Could you check a few things on this model? Use its own coordinates, in mm. Face numbers are marked on the shaded views. A direction names the side the tool comes from. Give positions to 0.01 mm unless a question says otherwise; leave off trailing zeros. Loops run counter-clockwise (first coordinate to the right, second up) from the corner with the lowest first, then second, coordinate; pieces in that order, holes last. Notation, with made-up numbers: (21, -8) -> (63, -8) arc R19 cw to (63, 24) -> close; hole circle Ø2 at (24, 27.25). An arc over 180 degrees is marked (long way). Put each result on its own line as item: value.
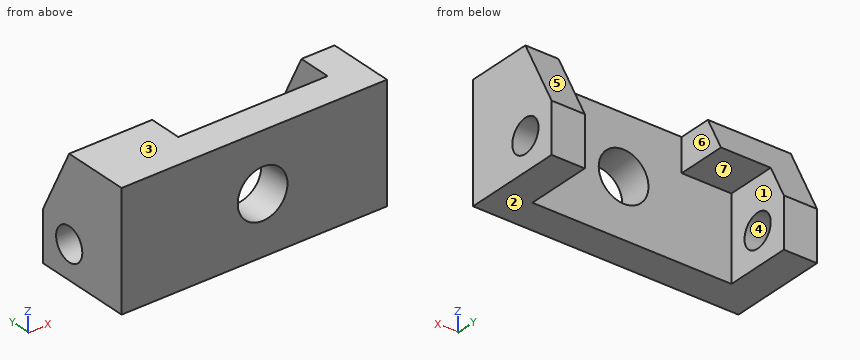
```python
from build123d import *

# Parameters (mm, degrees)
SKETCH1_W           = 80
SKETCH1_H           = 35
BOSS_EXTRUDE1_DEPTH = 30
CUT_EXTRUDE1_DEPTH  = 20
CUT_EXTRUDE2_DEPTH  = 81
SKETCH4_R           = 5
CUT_EXTRUDE4_DEPTH  = 81
SKETCH5_R           = 7.5
CUT_EXTRUDE5_DEPTH  = 11


with BuildPart() as part:
    # Sketch1 → Boss-Extrude1 (new body)
    with BuildSketch(Plane(origin=(0, 0, 0), x_dir=(1, 0, 0), z_dir=(0, 1, 0))):
        with Locations((40, 17.5)):
            Rectangle(SKETCH1_W, SKETCH1_H)
    extrude(amount=BOSS_EXTRUDE1_DEPTH)

    # Sketch2 → Cut-Extrude1 (cut)
    with BuildSketch(Plane(origin=(0, 30, 0), x_dir=(1, 0, 0), z_dir=(0, 1, 0))):
        Polygon((10, 35), (10, 10.002355001), (25, 10.002355001), (25, 0), (70, 0), (70, 35), align=None)
    extrude(amount=-CUT_EXTRUDE1_DEPTH, mode=Mode.SUBTRACT)

    # Sketch3 → Cut-Extrude2 (cut, through all)
    with BuildSketch(Plane.ZY):
        Polygon((0, 30), (0, 20), (-20, 30), align=None)
    extrude(amount=-CUT_EXTRUDE2_DEPTH, mode=Mode.SUBTRACT)

    # Sketch4 → Cut-Extrude4 (cut, through all)
    with BuildSketch(Plane(origin=(80, 0, 0), x_dir=(0, 0, -1), z_dir=(1, 0, 0))):
        with Locations((25, 20)):
            Circle(SKETCH4_R)
    extrude(amount=-CUT_EXTRUDE4_DEPTH, mode=Mode.SUBTRACT)

    # Sketch5 → Cut-Extrude5 (cut, through all)
    with BuildSketch(Plane(origin=(0, 10, 0), x_dir=(1, 0, 0), z_dir=(0, 1, 0))):
        with Locations((42.5, 17.5)):
            Circle(SKETCH5_R)
    extrude(amount=-CUT_EXTRUDE5_DEPTH, mode=Mode.SUBTRACT)


solid = part.part
```
1. If we section it at A-A (x = 48.5): List the corners of the cut face in (y, z) for me, then the cut area to 3 significant figures.
Recorded:
outline: (0, -35) -> (10, -35) -> (10, -22) -> (0, -22) -> close; (0, -13) -> (10, -13) -> (10, 0) -> (0, 0) -> close
area: 260 mm^2
2. I'm going to push flat-ended pins straight in: pin 1 (6 mm diameter, centred on x = 70.5, z = -30.5, fed in from -Y); pin 2 (5 mm diameter, centred on x = 48, z = -8, fed in from +Y); pin 3 (10 mm diameter, centred on x = 8, z = -14, fed in from +Y). Where does each tip first touch, or does it pass through?
Recorded:
pin 1: stops at y = 0
pin 2: stops at y = 10
pin 3: stops at y = 29.5
3. If we section it at B-B (y = 24): List the corners of the cut face in (x, z) for me, then the cut area to 3 significant figures.
Recorded:
outline: (0, -35) -> (10, -35) -> (10, -28) -> (0, -28) -> close; (0, -22) -> (10, -22) -> (10, -10) -> (25, -10) -> (25, -8) -> (0, -8) -> close; (70, -35) -> (80, -35) -> (80, -28) -> (70, -28) -> close; (70, -22) -> (80, -22) -> (80, -8) -> (70, -8) -> close
area: 450 mm^2
4. If we section it at C-C (z = -17.5): List the corners of the cut face in (x, y) for me, then the cut area to 4 significant figures.
Recorded:
outline: (0, 0) -> (35, 0) -> (35, 10) -> (10, 10) -> (10, 28.75) -> (0, 28.75) -> close; (50, 0) -> (80, 0) -> (80, 28.75) -> (70, 28.75) -> (70, 10) -> (50, 10) -> close
area: 1,025 mm^2
5. If we section it at D-D (z = -32): List the corners of the cut face in (x, y) for me.
Recorded:
outline: (0, 0) -> (80, 0) -> (80, 30) -> (70, 30) -> (70, 10) -> (10, 10) -> (10, 30) -> (0, 30) -> close
6. Thinking about a two-plate mould opening in Z: for the marked faces 1, 2, 3 and 4, which applies, pulls with the +Z half, pulls with the -Z half, needs draft (parallel to the pull), parting line crosses it, or undercut?
Recorded:
face 1: needs draft
face 2: pulls with the -Z half
face 3: pulls with the +Z half
face 4: undercut
7. For the marked faces 5, 6 and 7, which set-ups out of +Z, -Z, +X, -X, +Y, -Y let a thin tool reach every point of the face, with its end or its side?
Recorded:
face 5: +Z, +X, -X, +Y
face 6: +Z, -Z, +Y
face 7: -Z, +Y
8. I need wall thicknesses on line 1 (Z direction, x = 42.5, y = 6.5); line 2 (Y direction, x = 5, z = -25); line 3 (X direction, y = 20.5, z = -30.5). Which ranges of each line are inside material? Lowest first, please.
Recorded:
line 1: z = -35 to -25, -10 to 0
line 2: y = 0 to 15, 25 to 30
line 3: x = 0 to 10, 70 to 80
